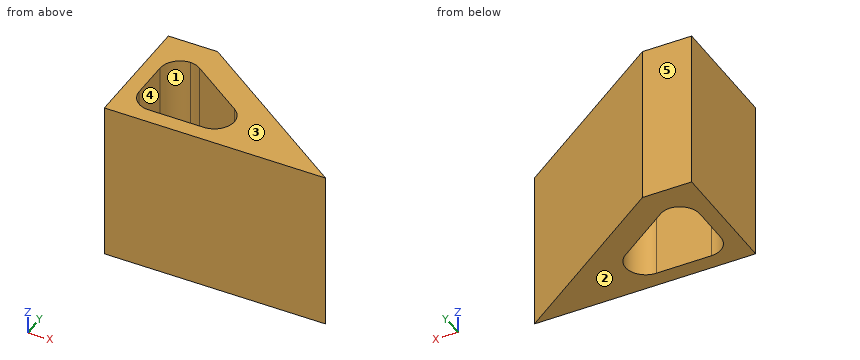
```python
from build123d import *

# Parameters (mm, degrees)
CROQUIS1_W              = 70
CROQUIS1_H              = 50.8
SALIENTE_EXTRUIR1_DEPTH = 38.1
CORTAR_EXTRUIR5_DEPTH   = 95.510581418
CORTAR_EXTRUIR6_DEPTH   = 95.510581418


with BuildPart() as part:
    # Croquis1 → Saliente-Extruir1 (new body)
    with BuildSketch(Plane(origin=(0, 0, 0), x_dir=(1, 0, 0), z_dir=(0, 1, 0))):
        with Locations((35, 0)):
            Rectangle(CROQUIS1_W, CROQUIS1_H)
    extrude(amount=SALIENTE_EXTRUIR1_DEPTH)

    # Croquis2 → Cortar-Extruir5 (cut, through all)
    with BuildSketch(Plane.XY.offset(25.4)):
        Polygon((70, 0), (15.587560943, 38.1), (70, 38.1), align=None)
    extrude(amount=-CORTAR_EXTRUIR5_DEPTH, mode=Mode.SUBTRACT)

    # Croquis3 → Cortar-Extruir6 (cut, through all)
    with BuildSketch(Plane.XY.offset(25.4)):
        with BuildLine():
            ThreePointArc((11.206511661, 30.09837862), (6.809424544, 28.189107402), (5, 23.75))
            Line((5, 23.75), (5, 11.35))
            ThreePointArc((5, 11.35), (6.859871939, 6.859871939), (11.35, 5))
            Line((11.35, 5), (28.772058606, 5))
            ThreePointArc((28.772058606, 5), (34.828161244, 9.440518173), (32.414268977, 16.551615481))
            Line((32.414268977, 16.551615481), (14.705233694, 28.951615481))
            ThreePointArc((14.705233694, 28.951615481), (13.040811255, 29.784140775), (11.206511661, 30.09837862))
        make_face()
    extrude(amount=-CORTAR_EXTRUIR6_DEPTH, mode=Mode.SUBTRACT)


solid = part.part
```
For this review, take the finished solid that the model builds, in its own axes (mm). Face numbers are marked on the shaded views. A direction names the side the tool comes from. Round coordinates to 2 decimals unless told otherwise and drop trailing zeros. Write each loop counter-clockwise with the first axis right and the second up, starting at its lowest first coordinate (ties: lowest second). Pieces come first, ordered by that corner, then holes. Notation, with made-up numbers: (-17.5, 64.25) -> (-0.5, 64.25) arc R38 cw to (-0.5, 103.25) -> close; hole circle Ø8 at (35.5, -26.75). An arc over 180 degrees is marked (long way). One line per question, with ' | ' between items. Start each with the question number.
1) For pin 1 Ø5 at (x, z) = (38, 14.5) entering from +Y; pin 2 Ø10 at (y, z) = (32, -4) entering from +X; pin 3 Ø10 at (y, z) = (19.5, -9) entering from +X; pin 4 Ø1 at (y, z) = (20.5, -14) entering from -X, all flat-tipped, find the tip position at first contact; note any pin that passes through.
2) Add section C-C (y = 19.5). Write out the cut boundary in (x, z), and give its area (3 significant figures).
3) Machinability: for the marked faces 1 and 2, which of the approach directions +Z, -Z, +X, -X, +Y, -Y give a long, thin tool a straight path to every point of the face, cutting with its end or side? Answer none if there is none.
4) Add section A-A (x = 23.5). Write out the cut boundary in (y, z), and give its area (3 significant figures).
5) Wall thickness on line 1 along Y through (x, z) = (21, -20); line 2 along X through (y, z) = (13, 21); line 3 along X through (y, z) = (14, -21.5): over which ranges is each line inside the solid? List them lowest first.
6) Mouldability with a two-part tool opening along Y and no side actions: class the marked faces 3, 4 and 5 as +Y half, -Y half, draft (parallel to the pull), parting line (faces both ways), or undercut.
7) Add section D-D (y = 34.5). Write out the cut boundary in (x, z), and give its area (3 significant figures).
8) Add section B-B (z = -12). Write out the cut boundary in (x, y), and give its area (3 significant figures).
Reported:
1) pin 1: stops at y = 24.16 | pin 2: stops at x = 31.44 | pin 3: stops at x = 49.29 | pin 4: stops at x = 0
2) outline: (0, -25.4) -> (5, -25.4) -> (5, 25.4) -> (0, 25.4) -> close; (28.2, -25.4) -> (42.15, -25.4) -> (42.15, 25.4) -> (28.2, 25.4) -> close | area: 963 mm²
3) face 1: +Z, -Z | face 2: -Z, +X, -X, +Y, -Y
4) outline: (0, -25.4) -> (5, -25.4) -> (5, 25.4) -> (0, 25.4) -> close; (22.79, -25.4) -> (32.56, -25.4) -> (32.56, 25.4) -> (22.79, 25.4) -> close | area: 750 mm²
5) line 1: y = 0 to 5, 24.54 to 34.31 | line 2: x = 0 to 5, 34.9 to 51.43 | line 3: x = 0 to 5, 34.54 to 50.01
6) face 3: draft | face 4: undercut | face 5: +Y half
7) outline: (0, -25.4) -> (20.73, -25.4) -> (20.73, 25.4) -> (0, 25.4) -> close | area: 1,050 mm²
8) outline: (0, 0) -> (70, 0) -> (15.59, 38.1) -> (0, 38.1) -> close; hole (5, 11.35) arc R6.35 ccw to (11.35, 5) -> (28.77, 5) arc R6.35 ccw to (32.41, 16.55) -> (14.71, 28.95) arc R6.35 ccw to (11.21, 30.1) arc R6.35 ccw to (5, 23.75) -> close | area: 1,070 mm²
